Geometry check sheet. Reference: the model listing, model coordinates, mm. A direction names the side the tool comes from. Give positions to 0.01 mm unless a question says otherwise; leave off trailing zeros. Order: outer loops, then holes, each group sorted by start corner. A loop starts at its lowest first (then second) coordinate and runs counter-clockwise, first axis right, second up.
```python
from build123d import *

# Parameters (mm, degrees)
SKETCH1_R           = 10
BOSS_EXTRUDE1_DEPTH = 142.050008
BOSS_EXTRUDE2_DEPTH = 3
SKETCH4_W           = 50.8
SKETCH4_H           = 3
BOSS_EXTRUDE3_DEPTH = 6.35
SKETCH5_R           = 6
CUT_EXTRUDE1_DEPTH  = 3


with BuildPart() as part:
    # Sketch1 → Boss-Extrude1 (new body)
    with BuildSketch(Plane(origin=(0, 0, 0), x_dir=(1, 0, 0), z_dir=(0, 1, 0))):
        Circle(SKETCH1_R)
    extrude(amount=BOSS_EXTRUDE1_DEPTH)

    # Sketch3 → Boss-Extrude2 (add)
    with BuildSketch(Plane.XZ):
        with BuildLine():
            Line((-0.9, 15.75), (0.9, 15.75))
            Line((0.9, 15.75), (0.9, 9.354806465))
            ThreePointArc((0.9, 9.354806465), (0, 9.398), (-0.9, 9.354806465))
            Line((-0.9, 9.354806465), (-0.9, 15.75))
        make_face()
    extrude(amount=-BOSS_EXTRUDE2_DEPTH)

    # Sketch4 → Boss-Extrude3 (add)
    with BuildSketch(Plane(origin=(0, 142.050008, 0), x_dir=(1, 0, 0), z_dir=(0, 1, 0))):
        Rectangle(SKETCH4_W, SKETCH4_H)
    extrude(amount=-BOSS_EXTRUDE3_DEPTH)

    # Sketch5 → Cut-Extrude1 (cut)
    with BuildSketch(Plane.XZ):
        Circle(SKETCH5_R)
    extrude(amount=-CUT_EXTRUDE1_DEPTH, mode=Mode.SUBTRACT)


solid = part.part
```
Q1. Cross-section at B-B, the plane x = 16. Record the boundary of the cut face in (y, z).
Q2. Cross-section at C-C, the plane y = 91.5. Record the boundary of the cut face in (x, z), and give its area (3 significant figures).
Q3. Cross-section at D-D, the plane z = 8. Record the boundary of the cut face in (x, y).
Q4. Release check for a two-part mould opening along X. For faces 4 (the face through (-6, 1, 0)), 5 (the face through (18, 139, 1.5)), 6 (the face through (-2.17, 70.03, 9.76)), 7 (the face through (0, 3, 0)) record: pulls with the +X half, pulls with the -X half, needs draft (parallel to the pull), parting line crosses it, or undercut.
Q5. Thickness scan on L1, parallel to Z at x = 0, y = 1.9; L2, parallel to Y at x = -4, z = 0; L3, parallel to Y at x = -13, z = 1. Record the ranges inside material, lowest first.
Q6. Gauge pin test, flat ends, axial feed: P1, Ø3, axis at y = 73, z = -7, coming from the +X side; P2, Ø1.5, axis at x = -14, z = -0.5, coming from the -Y side; P3, Ø0.9, axis at x = 0, z = 12.5, coming from the +Y side; P4, Ø1.5, axis at x = -11.5, y = 66.5, coming from the -Z side. Record the tip position at first contact, or that the pin passes through.
Q7. Access from +Z, -Z, +X, -X, +Y, -Y to the whole of each face (thin tool, end or side, straight path). Record for faces 1 (the face through (-18, 139, -1.5)), 2 (the face through (-0.9, 1, 13)), 3 (the face through (0.9, 1, 13)).
Q8. Cross-section at A-A, the plane z = 0. Record the boundary of the cut face in (x, y).
Answers follow:
1. outline: (135.7, -1.5) - (142.05, -1.5) - (142.05, 1.5) - (135.7, 1.5) - close
2. outline: circle Ø20 at (0, 0)
2. area: 314 mm2
3. outline: (-6, 0) - (6, 0) - (6, 142.05) - (-6, 142.05) - close
4. face 4: undercut
4. face 5: needs draft
4. face 6: parting line crosses it
4. face 7: undercut
5. L1: z = -10 to -6, 6 to 15.75
5. L2: y = 3 to 142.05
5. L3: y = 135.7 to 142.05
6. P1: stops at x = 8.35
6. P2: stops at y = 135.7
6. P3: stops at y = 3
6. P4: passes through
7. face 1: -Z, -X, +Y, -Y
7. face 2: +Z, -X, +Y, -Y
7. face 3: +Z, +X, +Y, -Y
8. outline: (-25.4, 135.7) - (-10, 135.7) - (-10, 0) - (-6, 0) - (-6, 3) - (6, 3) - (6, 0) - (10, 0) - (10, 135.7) - (25.4, 135.7) - (25.4, 142.05) - (-25.4, 142.05) - close
